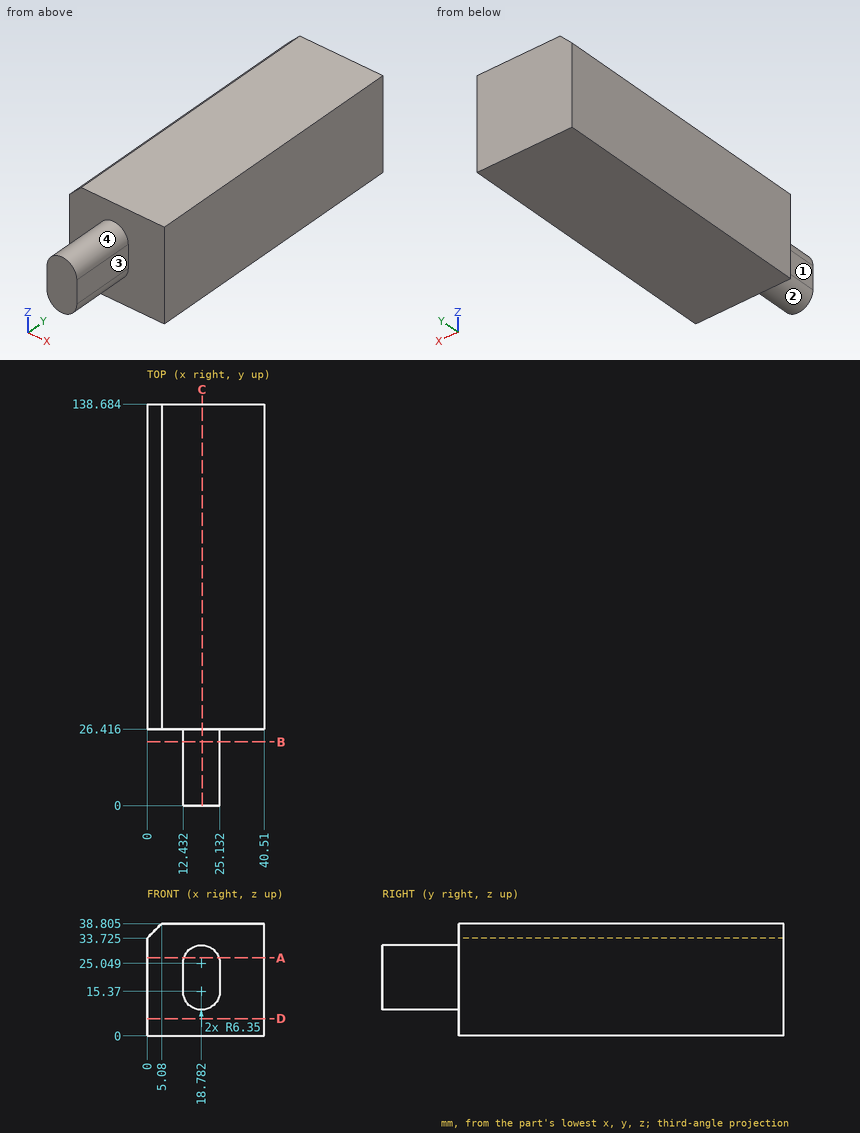
For this review, use the dimensioned drawing (mm, ordinates from the lowest corner) and the shaded views. A direction names the side the tool comes from. Give positions to 0.01 mm unless a question says otherwise; leave off trailing zeros. Write each loop counter-clockwise with the first axis right and the second up, starting at its lowest first coordinate (ties: lowest second). Pieces come first, ordered by that corner, then holes. Notation, with made-up numbers: M -26.75,-13 L -22.75,-13 A20 cw -22.75,14 Z; hole C 30.25,60 d10. An arc over 180 degrees is marked long. Answer as a JSON object with one key per item and string values. Group by question number.
Item 1: Consider section A-A on z = 27. Write out the cut boundary in (x, y) (1 decimal), plus the area to 3 significant figures.
Item 2: Consider section C-C on x = 19. Write out the cut boundary in (y, z) (1 decimal).
Item 3: Consider section D-D on z = 6. Write out the cut boundary in (x, y), plus the area to 3 significant figures.
Item 4: Consider section B-B on y = 22. Write out the cut boundary in (x, z).
Item 5: For pin 1 Ø3 at (y, z) = (12.5, 18) entering from +X; pin 2 Ø10 at (x, z) = (20.5, 24.5) entering from -Y; pin 3 Ø3 at (y, z) = (13.5, 22.5) entering from -X, all flat-tipped, find the tip position at first contact; note any pin that passes through.
Item 6: For probe 1 along Y at (x, z) = (30, 2); probe 2 along X at (y, z) = (7, 17); probe 3 along Z at (x, y) = (18, 22), list the stretches that pass through material, from the lowest coordinate up. Write a range as [from, to].
Item 7: Tool access review of the marked faces 1, 2, 3 and 4: name each direction out of +Z, -Z, +X, -X, +Y, -Y from which nothing blocks a thin tool from reaching the whole face with its end or side.
Check result:
{
 "1": {"outline": "M 0,26.4 L 12.7,26.4 L 12.7,0 L 24.8,0 L 24.8,26.4 L 40.5,26.4 L 40.5,138.7 L 0,138.7 Z", "area": "4,870 mm^2"},
 "2": {"outline": "M 0,9 L 26.4,9 L 26.4,0 L 138.7,0 L 138.7,38.8 L 26.4,38.8 L 26.4,31.4 L 0,31.4 Z"},
 "3": {"outline": "M 0,26.42 L 40.51,26.42 L 40.51,138.68 L 0,138.68 Z", "area": "4,550 mm^2"},
 "4": {"outline": "M 12.43,15.37 A6.35 ccw 25.13,15.37 L 25.13,25.05 A6.35 ccw 12.43,25.05 Z"},
 "5": {"pin 1": "stops at x = 25.13", "pin 2": "stops at y = 0", "pin 3": "stops at x = 12.43"},
 "6": {"probe 1": "y = [26.42, 138.68]", "probe 2": "x = [12.43, 25.13]", "probe 3": "z = [9.07, 31.35]"},
 "7": {"face 1": "+Z, -Z, -X, -Y", "face 2": "-Z, -Y", "face 3": "+Z, -Z, +X, -Y", "face 4": "+Z, -Y"}
}
